Build history of the part. All positions in model axes, mm. A direction names the side the tool comes from. Round coordinates to 2 decimals unless told otherwise and drop trailing zeros. Order: outer loops, then holes, each group sorted by start corner. A loop starts at its lowest first (then second) coordinate and runs counter-clockwise, first axis right, second up. Notation, with made-up numbers: M 69,19.25 L 111,19.25 A18 cw 111,40.25 Z; hole C 39.5,1 d3. An arc over 180 degrees is marked long. One line per item, written item: value. Start each with the question number.
Item 1: Tool access for faces 1 (the cylindrical face through (-4.85, 1.01, 9.78)), 2 (the flat face through (0, 2, 0)), 3 (the flat face through (-14, -22.75, -6)), 4 (the flat face through (-14, -27, 3.35)), 5 (the flat face through (-13, -16, 0)): list every direction of +Z, -Z, +X, -X, +Y, -Y with a clear straight run to the whole face (end or side of a thin tool).
Item 2: Pin check, flat tips, straight feed: pin 1 (12 mm diameter, centred on x = 4.5, z = 9, fed in from -Y); pin 2 (0.6 mm diameter, centred on x = -14, z = 6, fed in from -Y). Stop position of each tip, or through.
Item 3: Band-saw the part on D-D, the plane x = -5. Write the cut outline in (y, z).
Item 4: Band-saw the part on A-A, the plane x = -14. Write the cut outline in (y, z), then the cut area to 3 significant figures.
Item 5: Probe L1, parallel to Z at x = -14, y = -24.55; L2, parallel to Y at x = 8.25, z = -2.25; L3, parallel to X at y = -20, z = 11.25. List the from-to ranges inside material, lowest first.
Item 6: Band-saw the part on C-C, the plane y = -12. Write the cut outline in (x, z), then the cut area to 3 significant figures.
Item 7: Band-saw the part on B-B, the plane z = 10.5. Write the cut outline in (x, y).
Item 8: Two-plate mould, pull along Z, no slides. Class faces 6 (the flat face through (-15, -15, 0)), 7 (the cylindrical face through (9.93, 1.01, -6.61)), 8 (the flat face through (-13.3, -7.6, -12)): +Z half, -Z half, draft (parallel to the pull), parting line (faces both ways), or undercut.
Autodesk Inventor part; units mm, degrees
ref_plane "РабПлоскость1" through (-96.45, -32.75, -191.5) normal (0, 1, 0) x (0, 0, 1)
ref_plane "YZ Plane" through (0, 0, 0) normal (1, 0, 0) x (0, 1, 0)
ref_plane "XZ Plane" through (0, 0, 0) normal (0, 1, 0) x (-1, 0, 0)
sketch "Эскиз1" plane through (0, 0, 0) normal (0, 1, 0) x (-1, 0, 0)
  line L0 (-15, -12) -> (15, -12)
  line L1 (15, -12) -> (15, 12)
  line L2 (15, 12) -> (-15, 12)
  line L3 (-15, 12) -> (-15, -12)
  line L4 (-15, -12) -> (15, 12) construction
  line L5 (15, -12) -> (-15, 12) construction
  point P0 (0, 0)
  dimension "d0" = 24
  dimension "d1" = 30
extrude "Выдавливание1" add sketch "Эскиз1" along normal blind 2
sketch "Эскиз2" plane through (0, 2, 0) normal (0, 1, 0) x (1, 0, 0)
  circle A0 centre (11.5163, 7.8272) radius 2
  circle A1 centre (11.5163, -7.8272) radius 2
  circle A2 centre (-4.4163, -7.8272) radius 2
  circle A3 centre (-4.4163, 7.8272) radius 2
  point P0 (0, 0)
extrude "Выдавливание2" cut sketch "Эскиз2" against normal blind 2
sketch "Эскиз3" plane through (0, 0, 0) normal (0, -1, 0) x (1, 0, 0)
  line L0 (15, -12) -> (-15, -12)
  line L1 (-15, 12) -> (15, 12)
  line L2 (-15, -12) -> (-13, -12)
  line L3 (-13, -12) -> (-13, 12)
  line L4 (-13, 12) -> (-15, 12)
  line L5 (-15, 12) -> (-15, -12)
  point P0 (0, 0)
  dimension "d6" = 2
ref_plane "РабПлоскость1" through (-96.45, -32.75, -191.5) normal (0, 1, 0) x (0, 0, 1)
extrude "Выдавливание3" add sketch "Эскиз3" along normal up to surface (32.75 mm away)
sketch "Эскиз4" plane through (-15, 2, -12) normal (-1, 0, 0) x (0, 0, 1)
  line L0 (15.35, -27.95) -> (20.15, -27.95)
  line L1 (20.15, -27.95) -> (20.15, -29.75)
  line L2 (20.15, -29.75) -> (15.35, -29.75)
  line L3 (15.35, -29.75) -> (15.35, -27.95)
  line L4 (15.35, -27.95) -> (20.15, -29.75) construction
  line L5 (20.15, -27.95) -> (15.35, -29.75) construction
  line L6 (3.85, -27.95) -> (8.65, -27.95)
  line L7 (8.65, -27.95) -> (8.65, -29.75)
  line L8 (3.85, -29.75) -> (3.85, -27.95)
  line L9 (3.85, -27.95) -> (8.65, -29.75) construction
  line L10 (8.65, -27.95) -> (3.85, -29.75) construction
  line L11 (8.65, -29.75) -> (3.85, -29.75)
  line L12 (24, -2) -> (24, -34.75)
  line L13 (24, -34.75) -> (-0.0211, -34.75)
  line L14 (0, 0) -> (0, -34.75)
  line L15 (24, -34.75) -> (24, 0)
  line L16 (0, 0) -> (24, 0)
  line L17 (0, 0) -> (0, -34.75)
  line L18 (24, -34.75) -> (0, -34.75)
  point P0 (12, -2)
  point P1 (17.75, -28.85)
  point P2 (6.25, -28.85)
  dimension "d9" = 4.8
  dimension "d10" = 1.8
  dimension "d13" = 4.8
  dimension "d14" = 1.8
  dimension "d15" = 5
  dimension "d16" = 5
  dimension "d17" = 3.85
  dimension "d18" = 3.85
extrude "Выдавливание5" cut sketch "Эскиз4" against normal blind 10 contours L0 L1 L2 L3 | L6 L7 L11 L8
sketch "Эскиз5" plane through (-15, -32.75, -12) normal (0, -1, 0) x (1, 0, 0)
  circle A0 centre (1, 6.25) radius 1
  circle A1 centre (1, 17.75) radius 1
  point P0 (15, 12)
extrude "Выдавливание7" cut sketch "Эскиз5" against normal blind 10
properties part number "крепление энкодера"
Output:
1. face 1: +Y, -Y
1. face 2: +Z, -Z, +X, -X, +Y
1. face 3: -Y
1. face 4: +X, -X
1. face 5: +Z, -Z, +X, -Y
2. pin 1: stops at y = 0
2. pin 2: stops at y = -22.75
3. outline: M 0,-12 L 2,-12 L 2,-9.74 L 0,-9.74 Z; M 0,-5.91 L 2,-5.91 L 2,5.91 L 0,5.91 Z; M 0,9.74 L 2,9.74 L 2,12 L 0,12 Z
4. outline: M -32.75,-12 L 2,-12 L 2,12 L -32.75,12 L -32.75,6.75 L -27.75,6.75 L -27.75,8.15 L -25.95,8.15 L -25.95,6.75 L -22.75,6.75 L -22.75,4.75 L -25.95,4.75 L -25.95,3.35 L -27.75,3.35 L -27.75,4.75 L -32.75,4.75 L -32.75,-4.75 L -27.75,-4.75 L -27.75,-3.35 L -25.95,-3.35 L -25.95,-4.75 L -22.75,-4.75 L -22.75,-6.75 L -25.95,-6.75 L -25.95,-8.15 L -27.75,-8.15 L -27.75,-6.75 L -32.75,-6.75 Z
4. area: 784 mm²
5. L1: z = -12 to -6.75, -4.75 to 4.75, 6.75 to 12
5. L2: y = 0 to 2
5. L3: x = -15 to -13
6. outline: M -15,-12 L -13,-12 L -13,12 L -15,12 Z
6. area: 48.0 mm²
7. outline: M -15,-32.75 L -13,-32.75 L -13,0 L 15,0 L 15,2 L -15,2 Z
8. face 6: draft
8. face 7: undercut
8. face 8: -Z half
